from build123d import *

# Parameters (mm, degrees)
DIAL_PROFILE_SKETCH_R        = 19.1
DIAL_PROFILE_EXTRUSION_DEPTH = 6
BOSS_EXTRUDE1_START          = 5
SOCKET_TOP_SKETCH_R          = 19.1
BOSS_EXTRUDE1_DEPTH          = 5
CHAMFER1_SIZE                = 0.5


with BuildPart() as part:
    # Dial Profile Sketch → Dial Profile Extrusion (new body)
    with BuildSketch(Plane.XY):
        Circle(DIAL_PROFILE_SKETCH_R)
        with BuildLine():
            ThreePointArc((-0.85, 15.076057177), (0, 14.742572316), (0.85, 15.076057177))
            ThreePointArc((0.85, 15.076057177), (1.892531827, 14.98093199), (2.925967271, 14.813801522))
            ThreePointArc((2.925967271, 14.813801522), (3.666328646, 14.279407297), (4.572558645, 14.391028714))
            ThreePointArc((4.572558645, 14.391028714), (5.558680746, 14.039624937), (6.518085258, 13.620740236))
            ThreePointArc((6.518085258, 13.620740236), (7.102288379, 12.919014601), (8.007806614, 12.80175899))
            ThreePointArc((8.007806614, 12.80175899), (8.87555731, 12.216156615), (9.700647976, 11.571837747))
            ThreePointArc((9.700647976, 11.571837747), (10.091985213, 10.746872706), (10.939894643, 10.408107667))
            ThreePointArc((10.939894643, 10.408107667), (11.634749966, 9.625102245), (12.273683305, 8.795834135))
            ThreePointArc((12.273683305, 8.795834135), (12.4475655, 7.899465274), (13.184588857, 7.360476661))
            ThreePointArc((13.184588857, 7.360476661), (13.662888492, 6.429267303), (14.075517973, 5.467155915))
            ThreePointArc((14.075517973, 5.467155915), (14.021019468, 4.555705386), (14.600846863, 3.850359837))
            ThreePointArc((14.600846863, 3.850359837), (14.832537486, 2.82945785), (14.99293608, 1.794956182))
            ThreePointArc((14.99293608, 1.794956182), (14.713481217, 0.925693775), (15.099679963, 0.098310743))
            ThreePointArc((15.099679963, 0.098310743), (15.070203599, -0.948136845), (14.968292873, -1.990027249))
            ThreePointArc((14.968292873, -1.990027249), (14.481440829, -2.762482581), (14.649744639, -3.659915576))
            ThreePointArc((14.649744639, -3.659915576), (14.360953396, -4.666156615), (14.003136776, -5.64996995))
            ThreePointArc((14.003136776, -5.64996995), (13.339478254, -6.277081996), (13.27931198, -7.188175939))
            ThreePointArc((13.27931198, -7.188175939), (12.749351675, -8.090984604), (12.158112095, -8.954904259))
            ThreePointArc((12.158112095, -8.954904259), (11.359347202, -9.397269265), (11.074491312, -10.264776772))
            ThreePointArc((11.074491312, -10.264776772), (10.3366613, -11.007426274), (9.549148516, -11.697169))
            ThreePointArc((9.549148516, -11.697169), (8.665466588, -11.926991544), (8.173819626, -12.696403929))
            ThreePointArc((8.173819626, -12.696403929), (7.274480479, -13.232230869), (6.340176817, -13.704457593))
            ThreePointArc((6.340176817, -13.704457593), (5.427102839, -13.707297081), (4.759556791, -14.330269333))
            ThreePointArc((4.759556791, -14.330269333), (3.755217296, -14.625605733), (2.732828491, -14.850644714))
            ThreePointArc((2.732828491, -14.850644714), (1.847734259, -14.62632273), (1.046233499, -15.063711212))
            ThreePointArc((1.046233499, -15.063711212), (0, -15.1), (-1.046233499, -15.063711212))
            ThreePointArc((-1.046233499, -15.063711212), (-1.847734259, -14.62632273), (-2.732828491, -14.850644714))
            ThreePointArc((-2.732828491, -14.850644714), (-3.755217296, -14.625605733), (-4.759556791, -14.330269333))
            ThreePointArc((-4.759556791, -14.330269333), (-5.427102839, -13.707297081), (-6.340176817, -13.704457593))
            ThreePointArc((-6.340176817, -13.704457593), (-7.274480479, -13.232230869), (-8.173819626, -12.696403929))
            ThreePointArc((-8.173819626, -12.696403929), (-8.665466588, -11.926991544), (-9.549148516, -11.697169))
            ThreePointArc((-9.549148516, -11.697169), (-10.3366613, -11.007426274), (-11.074491312, -10.264776772))
            ThreePointArc((-11.074491312, -10.264776772), (-11.359347202, -9.397269265), (-12.158112095, -8.954904259))
            ThreePointArc((-12.158112095, -8.954904259), (-12.749351675, -8.090984604), (-13.27931198, -7.188175939))
            ThreePointArc((-13.27931198, -7.188175939), (-13.339478254, -6.277081996), (-14.003136776, -5.64996995))
            ThreePointArc((-14.003136776, -5.64996995), (-14.360953396, -4.666156615), (-14.649744639, -3.659915576))
            ThreePointArc((-14.649744639, -3.659915576), (-14.481440829, -2.762482581), (-14.968292873, -1.990027249))
            ThreePointArc((-14.968292873, -1.990027249), (-15.070203599, -0.948136845), (-15.099679963, 0.098310743))
            ThreePointArc((-15.099679963, 0.098310743), (-14.713481217, 0.925693775), (-14.99293608, 1.794956182))
            ThreePointArc((-14.99293608, 1.794956182), (-14.832537486, 2.82945785), (-14.600846863, 3.850359837))
            ThreePointArc((-14.600846863, 3.850359837), (-14.021019468, 4.555705386), (-14.075517973, 5.467155915))
            ThreePointArc((-14.075517973, 5.467155915), (-13.662888492, 6.429267303), (-13.184588857, 7.360476661))
            ThreePointArc((-13.184588857, 7.360476661), (-12.4475655, 7.899465274), (-12.273683305, 8.795834135))
            ThreePointArc((-12.273683305, 8.795834135), (-11.634749966, 9.625102245), (-10.939894643, 10.408107667))
            ThreePointArc((-10.939894643, 10.408107667), (-10.091985213, 10.746872706), (-9.700647976, 11.571837747))
            ThreePointArc((-9.700647976, 11.571837747), (-8.87555731, 12.216156615), (-8.007806614, 12.80175899))
            ThreePointArc((-8.007806614, 12.80175899), (-7.102288379, 12.919014601), (-6.518085258, 13.620740236))
            ThreePointArc((-6.518085258, 13.620740236), (-5.558680746, 14.039624937), (-4.572558645, 14.391028714))
            ThreePointArc((-4.572558645, 14.391028714), (-3.666328646, 14.279407297), (-2.925967271, 14.813801522))
            ThreePointArc((-2.925967271, 14.813801522), (-1.892531827, 14.98093199), (-0.85, 15.076057177))
        make_face(mode=Mode.SUBTRACT)
    extrude(amount=DIAL_PROFILE_EXTRUSION_DEPTH)

    # Socket Top Sketch → Boss-Extrude1 (add)
    with BuildSketch(Plane(origin=(0, 0, 0), x_dir=(-1, 0, 0), z_dir=(0, 0, -1)).offset(BOSS_EXTRUDE1_START)):
        Circle(SOCKET_TOP_SKETCH_R)
        with BuildLine():
            Line((-1.626412403, 12.183897348), (-3.218122555, 6.940820202))
            ThreePointArc((-3.218122555, 6.940820202), (-3.675, 6.365286718), (-4.401865341, 6.257385986))
            Line((-4.401865341, 6.257385986), (-9.738358419, 7.500463132))
            ThreePointArc((-9.738358419, 7.500463132), (-10.464716593, 8.172122942), (-10.258132896, 9.139617786))
            ThreePointArc((-10.258132896, 9.139617786), (-6.86953244, 11.898379211), (-2.786074736, 13.453612576))
            ThreePointArc((-2.786074736, 13.453612576), (-1.844907774, 13.148771884), (-1.626412403, 12.183897348))
        make_face(mode=Mode.SUBTRACT)
        Polygon((0, 7.332348419), (-6.35, 3.666174209), (-6.35, -3.666174209), (0, -7.332348419), (6.35, -3.666174209), (6.35, 3.666174209), align=None, mode=Mode.SUBTRACT)
        with BuildLine():
            Line((3.218122555, 6.940820202), (1.626412403, 12.183897348))
            ThreePointArc((1.626412403, 12.183897348), (1.844907774, 13.148771884), (2.786074736, 13.453612576))
            ThreePointArc((2.786074736, 13.453612576), (6.86953244, 11.898379211), (10.258132896, 9.139617786))
            ThreePointArc((10.258132896, 9.139617786), (10.464716593, 8.172122942), (9.738358419, 7.500463132))
            Line((9.738358419, 7.500463132), (4.401865341, 6.257385986))
            ThreePointArc((4.401865341, 6.257385986), (3.675, 6.365286718), (3.218122555, 6.940820202))
        make_face(mode=Mode.SUBTRACT)
        with BuildLine():
            Line((7.619987896, 0.683434216), (11.364770822, 4.683434216))
            ThreePointArc((11.364770822, 4.683434216), (12.309624367, 4.976648942), (13.044207632, 4.31399479))
            ThreePointArc((13.044207632, 4.31399479), (13.73906488, 0), (13.044207632, -4.31399479))
            ThreePointArc((13.044207632, -4.31399479), (12.309624367, -4.976648942), (11.364770822, -4.683434216))
            Line((11.364770822, -4.683434216), (7.619987896, -0.683434216))
            ThreePointArc((7.619987896, -0.683434216), (7.35, 0), (7.619987896, 0.683434216))
        make_face(mode=Mode.SUBTRACT)
        with BuildLine():
            Line((4.401865341, -6.257385986), (9.738358419, -7.500463132))
            ThreePointArc((9.738358419, -7.500463132), (10.464716593, -8.172122942), (10.258132896, -9.139617786))
            ThreePointArc((10.258132896, -9.139617786), (6.86953244, -11.898379211), (2.786074736, -13.453612576))
            ThreePointArc((2.786074736, -13.453612576), (1.844907774, -13.148771884), (1.626412403, -12.183897348))
            Line((1.626412403, -12.183897348), (3.218122555, -6.940820202))
            ThreePointArc((3.218122555, -6.940820202), (3.675, -6.365286718), (4.401865341, -6.257385986))
        make_face(mode=Mode.SUBTRACT)
        with BuildLine():
            Line((-3.218122555, -6.940820202), (-1.626412403, -12.183897348))
            ThreePointArc((-1.626412403, -12.183897348), (-1.844907774, -13.148771884), (-2.786074736, -13.453612576))
            ThreePointArc((-2.786074736, -13.453612576), (-6.86953244, -11.898379211), (-10.258132896, -9.139617786))
            ThreePointArc((-10.258132896, -9.139617786), (-10.464716593, -8.172122942), (-9.738358419, -7.500463132))
            Line((-9.738358419, -7.500463132), (-4.401865341, -6.257385986))
            ThreePointArc((-4.401865341, -6.257385986), (-3.675, -6.365286718), (-3.218122555, -6.940820202))
        make_face(mode=Mode.SUBTRACT)
        with BuildLine():
            Line((-7.619987896, -0.683434216), (-11.364770822, -4.683434216))
            ThreePointArc((-11.364770822, -4.683434216), (-12.309624367, -4.976648942), (-13.044207632, -4.31399479))
            ThreePointArc((-13.044207632, -4.31399479), (-13.73906488, 0), (-13.044207632, 4.31399479))
            ThreePointArc((-13.044207632, 4.31399479), (-12.309624367, 4.976648942), (-11.364770822, 4.683434216))
            Line((-11.364770822, 4.683434216), (-7.619987896, 0.683434216))
            ThreePointArc((-7.619987896, 0.683434216), (-7.35, 0), (-7.619987896, -0.683434216))
        make_face(mode=Mode.SUBTRACT)
    extrude(amount=-BOSS_EXTRUDE1_DEPTH)

    # Chamfer1
    chamfer1_edges = [part.edges().sort_by_distance(p)[0] for p in [
        (-3.675, 6.365286718, -5),
        (-2.422267479, 9.562358775, -5),
        (-6.86953244, 11.898379211, -5),
        (-10.464716593, 8.172122942, -5),
        (-7.07011188, 6.878924559, -5),
        (-3.675, -6.365286718, -5),
        (-7.07011188, -6.878924559, -5),
        (-6.86953244, -11.898379211, -5),
        (-1.844907774, -13.148771884, -5),
        (-2.422267479, -9.562358775, -5),
        (-7.35, 0, -5),
        (-9.492379359, 2.683434216, -5),
        (-13.73906488, 0, -5),
        (-12.309624367, -4.976648942, -5),
        (-9.492379359, -2.683434216, -5),
        (3.675, 6.365286718, -5),
        (7.07011188, 6.878924559, -5),
        (6.86953244, 11.898379211, -5),
        (1.844907774, 13.148771884, -5),
        (2.422267479, 9.562358775, -5),
        (7.35, 0, -5),
        (9.492379359, -2.683434216, -5),
        (13.73906488, 0, -5),
        (12.309624367, 4.976648942, -5),
        (9.492379359, 2.683434216, -5),
        (3.675, -6.365286718, -5),
        (2.422267479, -9.562358775, -5),
        (6.86953244, -11.898379211, -5),
        (10.464716593, -8.172122942, -5),
        (7.07011188, -6.878924559, -5),
        (19.1, 0, -5),
        (1.844907774, -13.148771884, -5),
        (12.309624367, -4.976648942, -5),
        (10.464716593, 8.172122942, -5),
        (-3.175, 5.499261314, -5),
        (3.175, 5.499261314, -5),
        (6.35, 0, -5),
        (3.175, -5.499261314, -5),
        (-3.175, -5.499261314, -5),
        (-6.35, 0, -5),
        (-12.309624367, 4.976648942, -5),
        (-10.464716593, -8.172122942, -5),
        (-1.844907774, 13.148771884, -5),
    ]]
    chamfer(chamfer1_edges, length=CHAMFER1_SIZE - 0.0001)  # a hair under: the kernel refuses the full size


solid = part.part
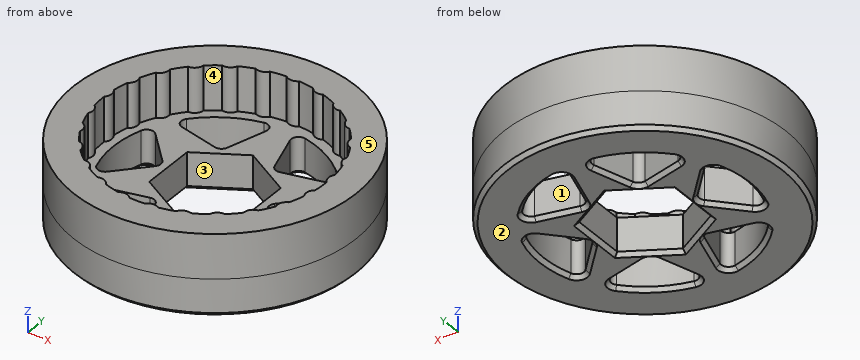
Here's how the part is built. I have some questions about the finished solid (model axes, mm). Face numbers are marked on the shaded views. A direction names the side the tool comes from. Coordinates: 2 decimals unless noted, no trailing zeros. Answer as CSV lines item,"result".
Item 1: For pin 1 (5 mm diameter, centred on y = -12.5, z = -2, fed in from -X); pin 2 (1 mm diameter, centred on x = -15, z = -3, fed in from -Y); pin 3 (1.5 mm diameter, centred on x = -12.5, z = -2, fed in from -Y), each with a flat end and sliding along its axis, tell me the tip position at first contact or that it passes through.
Results found:
pin 1,"x = -16.27"
pin 2,"y = -12.43"
pin 3,"y = -15.06"
Item 2: On a 3-axis mill with a long thin cutter (end or side, diameter ignored), from which of +Z, -Z, +X, -X, +Y, -Y can I reach the whole of each face in a straight line? I mean the marked faces 3, 4 and 5. Say none if no direction works.
Results found:
face 3,"+Z, -Z"
face 4,"+Z"
face 5,"+Z, +X, -X, +Y, -Y"
Item 3: We'd pull the mould along Y, two halves only. Please class the marked faces 1 and 2: +Y half, -Y half, draft (parallel to the pull), parting line (faces both ways), or undercut.
Results found:
face 1,"undercut"
face 2,"draft"
Item 4: Imagine slicing it at A-A on z = -4. Give the number of separate pieces and of enclosed holes in the cut face, plus the area to 3 significant figures.
Results found:
separate pieces,"1"
enclosed holes,"7"
area,"762 mm2"
Item 5: If I drill on line 1 (X direction, y = 3, z = -3.25); line 2 (Y direction, x = -5, z = -3.25); line 3 (X direction, y = -9.5, z = -2), over which ranges is the centre line in solid material (lowest first)?
Results found:
line 1,"-18.86 to -13.41, -9.79 to -6.35, 6.35 to 9.79, 13.41 to 18.86"
line 2,"-18.43 to -12.8, -6.4 to -4.45, 4.45 to 6.4, 12.8 to 18.43"
line 3,"-16.57 to -9.93, -2.44 to 2.44, 9.93 to 16.57"
